The figure shows three views and two pictorial views of one solid part (mm, origin at its lowest corner). Answer the questions. A direction names the side the tool comes from. Coordinates: 2 decimals unless noted, no trailing zeros. Order: outer loops, then holes, each group sorted by start corner. A loop starts at its lowest first (then second) coordinate and runs counter-clockwise, first axis right, second up. Notation, with made-up numbers: (13.5, -31.75) -> (66.5, -31.75) arc R19 ccw to (66.5, -21.75) -> close; hole circle Ø8 at (46, 30). An arc over 180 degrees is marked (long way). Write item = value, one per line.
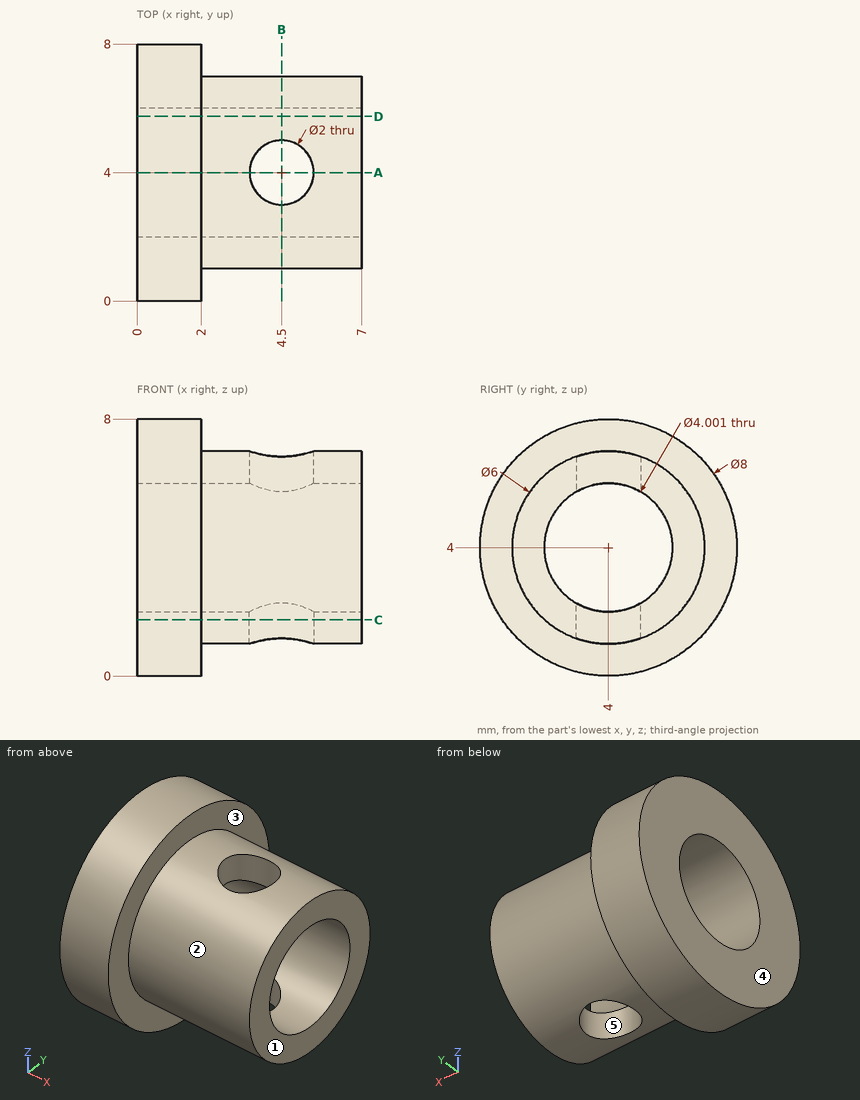
Q1. Section C-C, the plane z = 1.75 is taken. Give the vertices of the cut face in (x, y).
The answers:
outline = (0, 0.69) -> (2, 0.69) -> (2, 2.02) -> (7, 2.02) -> (7, 5.98) -> (2, 5.98) -> (2, 7.31) -> (0, 7.31) -> close; hole circle Ø2 at (4.5, 4)
Q2. A tool of negligible diameter and unlimited length cuts with its end or side. For the marked faces 1 and 2, from which of +Z, -Z, +X, -X, +Y, -Y can it reach the whole face along a straight path? Write none if from no direction.
The answers:
face_1 = +Z, -Z, +X, +Y, -Y
face_2 = +X
Q3. Find the intervals of material crossed by line 1 along X through (y, z) = (4, 1.8); line 2 along Z through (x, y) = (1.5, 4); line 3 along Y through (x, z) = (4.5, 6.2), in increasing order.
The answers:
line_1 = 0 to 3.5, 5.5 to 7
line_2 = 0 to 2, 6 to 8
line_3 = 1.96 to 3, 5 to 6.04
Q4. Section D-D, the plane y = 5.75 is taken. Give the vertices of the cut face in (x, z).
The answers:
outline = (0, 0.4) -> (2, 0.4) -> (2, 1.56) -> (7, 1.56) -> (7, 3.03) -> (0, 3.03) -> close; (0, 4.97) -> (7, 4.97) -> (7, 6.44) -> (2, 6.44) -> (2, 7.6) -> (0, 7.6) -> close
Q5. The mould has two halves that part along X. Classify the marked faces 3, 4 and 5: released by +X, released by -X, zero draft, split by the parting line, or undercut.
The answers:
face_3 = released by +X
face_4 = released by -X
face_5 = undercut
Q6. Section B-B, the plane x = 4.5 is taken. Give the vertices of the cut face in (y, z).
The answers:
outline = (3, 1.17) -> (3, 2.27) arc R2 cw to (3, 5.73) -> (3, 6.83) arc R3 ccw to start; (5, 1.17) arc R3 ccw to (5, 6.83) -> (5, 5.73) arc R2 cw to (5, 2.27) -> close
Q7. Each of these flat-tipped pins is pushed along its axis until it touches: pin 1 Ø1.2 at (x, y) = (4.5, 4) entering from +Z; pin 2 Ø4 at (x, y) = (3.5, 6.5) entering from -Z; pin 3 Ø2 at (x, y) = (3.5, 4) entering from -Z; pin 4 Ø3 at (x, y) = (4.5, 4) entering from +Z. Where does it stop, or does it pass through?
The answers:
pin_1 = through
pin_2 = 0.18
pin_3 = 1
pin_4 = 7
Q8. Section A-A, the plane y = 4 is taken. Give the vertices of the cut face in (x, z), plus the area to 3 significant figures.
The answers:
outline = (0, 0) -> (2, 0) -> (2, 1) -> (3.5, 1) -> (3.5, 2) -> (0, 2) -> close; (0, 6) -> (3.5, 6) -> (3.5, 7) -> (2, 7) -> (2, 8) -> (0, 8) -> close; (5.5, 1) -> (7, 1) -> (7, 2) -> (5.5, 2) -> close; (5.5, 6) -> (7, 6) -> (7, 7) -> (5.5, 7) -> close
area = 14.0 mm2
